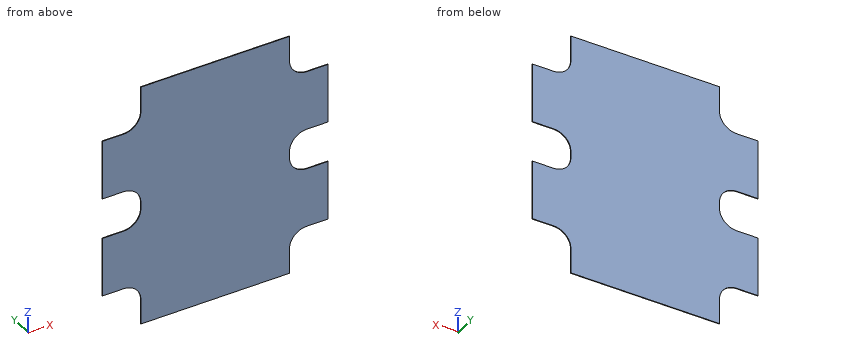
Autodesk Inventor part; units mm, degrees
ref_plane "YZ Plane" through (0, 0, 0) normal (1, 0, 0) x (0, 1, 0)
ref_plane "XZ Plane" through (0, 0, 0) normal (0, 1, 0) x (-1, 0, 0)
ref_plane "XY Plane" through (0, 0, 0) normal (0, 0, 1) x (1, 0, 0)
sketch "Sketch1" plane through (0, 0, 0) normal (0, 1, 0) x (-1, 0, 0)
  line L0 (-214, 360) -> (214, 360)
  line L1 (214, 360) -> (214, -360)
  line L2 (214, -360) -> (-214, -360)
  line L3 (-214, -360) -> (-214, 360)
  line L4 (-214, 360) -> (214, -360) construction
  line L5 (214, 360) -> (-214, -360) construction
  line L6 (214, -235) -> (325, -235)
  line L7 (325, -235) -> (325, -60)
  line L8 (325, -60) -> (214, -60)
  line L9 (214, -60) -> (214, -235)
  line L10 (214, 60) -> (325, 60)
  line L11 (325, 60) -> (325, 235)
  line L12 (325, 235) -> (214, 235)
  line L13 (214, 235) -> (214, 60)
  line L14 (0, 360) -> (0, 260) construction
  line L15 (0, 360) -> (100, 360) construction
  line L16 (-214, -235) -> (-325, -235)
  line L17 (-325, -235) -> (-325, -60)
  line L18 (-325, -60) -> (-214, -60)
  line L19 (-214, 60) -> (-325, 60)
  line L20 (-325, 60) -> (-325, 235)
  line L21 (-325, 235) -> (-214, 235)
  line L22 (-214, 235) -> (-214, 60)
  line L23 (-214, -60) -> (-214, -235)
  point P0 (0, 0)
  dimension "d0" = 720
  dimension "d1" = 428
  dimension "d4" = 111
  dimension "d5" = 175
  dimension "d6" = 125
  dimension "d7" = 111
  dimension "d8" = 175
  dimension "d9" = 125
  dimension "d10" = 100
  dimension "d11" = 90
extrude "Extrusion1" add sketch "Sketch1" along normal blind 2
fillet "Fillet1" radius 50 8 edges at (214, 1, -235) (214, 1, -60) (214, 1, 60) (214, 1, 235) (-214, 1, 60) (-214, 1, -60) (-214, 1, -235) (-214, 1, 235)
properties part number "Bottom Mounting Plate" material "Polycarbonate, Smoke"
Geometry: final body of the model. Coordinates: model frame, mm. Give positions to 0.01 mm unless a question says otherwise; leave off trailing zeros. Write each loop counter-clockwise with the first axis right and the second up, starting at its lowest first coordinate (ties: lowest second). Pieces come first, ordered by that corner, then holes. Notation, with made-up numbers: (72, -1.75) -> (112, -1.75) arc R27 ccw to (112, 17.25) -> close; hole circle Ø2 at (-2, 83.5). An arc over 180 degrees is marked (long way). Answer in a Markdown table with one row per item.
(1) Section query C-C on z = -45.5. Return loops of the section in (x, y).
Answers below:
| item | result |
|---|---|
| outline | (-228.79, 0) -> (228.79, 0) -> (228.79, 2) -> (-228.79, 2) -> close |
(2) Section query A-A on x = 227. Return loops of the section in (y, z), then the cut area to 3 significant figures.
Answers below:
| item | result |
|---|---|
| outline | (0, -251.37) -> (2, -251.37) -> (2, -43.63) -> (0, -43.63) -> close; (0, 43.63) -> (2, 43.63) -> (2, 251.37) -> (0, 251.37) -> close |
| area | 831 mm^2 |
(3) Section query D-D on z = 32. Return loops of the section in (x, y).
Answers below:
| item | result |
|---|---|
| outline | (-219.1, 0) -> (219.1, 0) -> (219.1, 2) -> (-219.1, 2) -> close |
(4) Ray query, line 1 along Z through (x, y) = (-292, 1.75); line 2 along X through (y, z) = (0.2, 294.5); line 3 along X through (y, z) = (1.35, -259.5). Return the intervals inside material, ascending. Write a range as [from, to].
Answers below:
| item | result |
|---|---|
| line 1 | [-235, -60], [60, 235] |
| line 2 | [-214, 214] |
| line 3 | [-220.99, 220.99] |
(5) Pin query (flat end, axial travel): pin 1 (0.6 mm diameter, centred on x = -288.5, y = 1, fed in from +Z); pin 2 (1 mm diameter, centred on y = 0.5, z = 304.5, fed in from -X); pin 3 (1 mm diameter, centred on y = 1.5, z = -332, fed in from +X). Return the tip coordinate at first contact, or that it passes through.
Answers below:
| item | result |
|---|---|
| pin 1 | z = 235 |
| pin 2 | x = -214 |
| pin 3 | x = 214 |
(6) Section query B-B on y = 1. Return loops of the section in (x, z).
Answers below:
| item | result |
|---|---|
| outline | (-325, -235) -> (-264, -235) arc R50 cw to (-214, -285) -> (-214, -360) -> (214, -360) -> (214, -285) arc R50 cw to (264, -235) -> (325, -235) -> (325, -60) -> (264, -60) arc R50 cw to (214, -10) -> (214, 10) arc R50 cw to (264, 60) -> (325, 60) -> (325, 235) -> (264, 235) arc R50 cw to (214, 285) -> (214, 360) -> (-214, 360) -> (-214, 285) arc R50 cw to (-264, 235) -> (-325, 235) -> (-325, 60) -> (-264, 60) arc R50 cw to (-214, 10) -> (-214, -10) arc R50 cw to (-264, -60) -> (-325, -60) -> close |
